Source: three-view drawing plus pictorial views. Frame: mm from the lowest corner of the part. Round coordinates to 2 decimals unless told otherwise and drop trailing zeros. Loops run counter-clockwise (first coordinate to the right, second up) from the corner with the lowest first, then second, coordinate; pieces in that order, holes last. Notation, with made-up numbers: (3, 3.5) -> (46, 3.5) arc R32 cw to (46, 31.5) -> close; hole circle Ø3 at (6.5, 69.5). An arc over 180 degrees is marked (long way). Answer as a JSON object with one key per item and string values. Group by question number.
Item 1: Material intervals for line 1 (Y direction, x = 7.5, z = 9); line 2 (X direction, y = 1.45, z = 5); line 3 (X direction, y = 2.85, z = 5), sorted ascending. Write a range as [from, to].
Item 2: Draft query along X for the marked faces 1, 2 and 3. Return one class per face: released by +X, released by -X, zero draft, split by the parting line, or undercut.
Item 3: Section query C-C on y = 0.7. Return loops of the section in (x, z).
Item 4: Section query B-B on z = 4.5. Return loops of the section in (x, y) (1 decimal).
Item 5: Section query D-D on x = 7.25. Return loops of the section in (y, z) (1 decimal), and give its area (3 significant figures).
Item 6: Section query A-A on x = 5. Return loops of the section in (y, z), and give its area (3 significant figures).
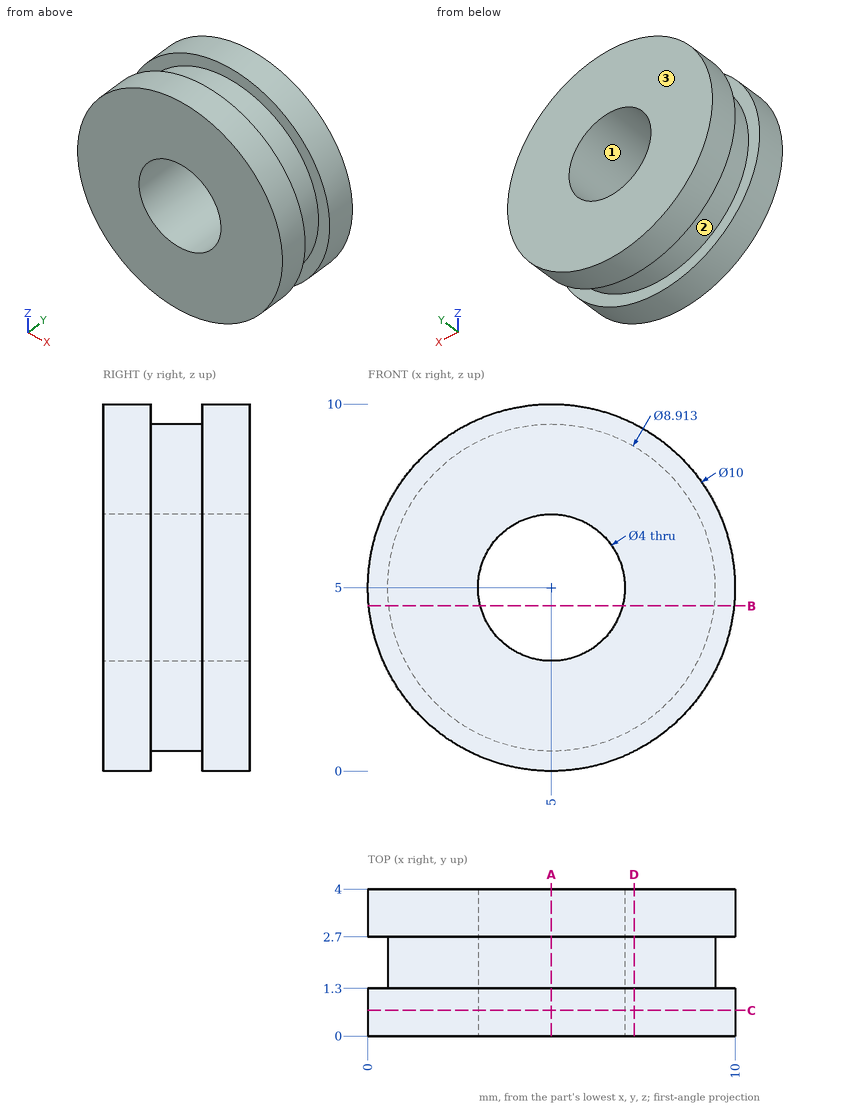
Solved:
{
 "1": {"line 1": "[0, 1.3], [2.7, 4]", "line 2": "[0.54, 3], [7, 9.46]", "line 3": "[0, 3], [7, 10]"},
 "2": {"face 1": "undercut", "face 2": "split by the parting line", "face 3": "zero draft"},
 "3": {"outline": "circle Ø10 at (5, 5); hole circle Ø4 at (5, 5)"},
 "4": {"outline": "(0, 0) -> (3.1, 0) -> (3.1, 4) -> (0, 4) -> (0, 2.7) -> (0.6, 2.7) -> (0.6, 1.3) -> (0, 1.3) -> close; (6.9, 0) -> (10, 0) -> (10, 1.3) -> (9.4, 1.3) -> (9.4, 2.7) -> (10, 2.7) -> (10, 4) -> (6.9, 4) -> close"},
 "5": {"outline": "(0, 0.5) -> (1.3, 0.5) -> (1.3, 1.2) -> (2.7, 1.2) -> (2.7, 0.5) -> (4, 0.5) -> (4, 9.5) -> (2.7, 9.5) -> (2.7, 8.8) -> (1.3, 8.8) -> (1.3, 9.5) -> (0, 9.5) -> close", "area": "34.0 mm²"},
 "6": {"outline": "(0, 0) -> (1.3, 0) -> (1.3, 0.54) -> (2.7, 0.54) -> (2.7, 0) -> (4, 0) -> (4, 3) -> (0, 3) -> close; (0, 7) -> (4, 7) -> (4, 10) -> (2.7, 10) -> (2.7, 9.46) -> (1.3, 9.46) -> (1.3, 10) -> (0, 10) -> close", "area": "22.5 mm²"}
}
